```python
from build123d import *

# Parameters (mm, degrees)
BOSS_EXTRUDE2_START = 5
SKETCH6_R           = 3
BOSS_EXTRUDE2_DEPTH = 5


with BuildPart() as part:
    # Sketch2 → Revolve1 (revolve)
    with BuildSketch(Plane.XY, mode=Mode.PRIVATE) as revolve1_sk:
        Polygon((-42.375, 0), (42.375, 0), (42.375, 3), (36.175, 3), (36.175, 3.5), (30.375, 3.5), (30.375, 5), (28.375, 5), (28.375, 6), (-17.625, 6), (-17.625, 5), (-32.375, 5), (-32.375, 3), (-42.375, 3), align=None)
    revolve(revolve1_sk.sketch.rotate(Axis((-42.375, 0, 0), (1, 0, 0)), 90), axis=Axis((-42.375, 0, 0), (1, 0, 0)))

    # Sketch6 → Boss-Extrude2 (add)
    with BuildSketch(Plane.ZY.offset(42.375).offset(BOSS_EXTRUDE2_START)):
        Circle(SKETCH6_R)
    extrude(amount=-BOSS_EXTRUDE2_DEPTH)


solid = part.part
```
CAD build for the part. Positions are in the model's coordinates, mm. A direction names the side the tool comes from. Round coordinates to 2 decimals unless told otherwise and drop trailing zeros. Write each loop counter-clockwise with the first axis right and the second up, starting at its lowest first coordinate (ties: lowest second). Pieces come first, ordered by that corner, then holes. Notation, with made-up numbers: (37.25, 58) -> (89.25, 58) arc R31 ccw to (89.25, 85) -> close; hole circle Ø7 at (20, 80). An arc over 180 degrees is marked (long way). Answer in a Markdown table with one row per item. Add a question column.
Item 1: Saw through at C-C, the plane x = 22.5. Write the cut outline in (y, z).
Item 2: Saw through at A-A, the plane z = 0. Write the cut outline in (x, y) (3 decimals), then the cut area to 3 significant figures.
Item 3: Which spindle directions (+Z, -Z, +X, -X, +Y, -Y) get a long thin tool onto all of the face, cutting with end or side? Do faces 1 (the face through (-32.375, -0.1, 3.3)), 2 (the face through (5.053, -1.802, 5.723)), 3 (the face through (30.375, 3.3, -2.2)). Say none if no direction does.
Item 4: Saw through at D-D, the plane z = 4.25. Write the cut outline in (x, y) (3 decimals), then the cut area to 3 significant figures.
Item 5: Drop flat-ended pins along their axis: pin 1 Ø1 at (x, y) = (0.5, -2) entering from -Z; pin 2 Ø6 at (y, z) = (3, -2.5) entering from -X (3 decimals); pin 3 Ø1.5 at (x, z) = (-24, 1.5) entering from +Y; pin 4 Ø6 at (x, z) = (-28.5, -4) entering from -Y. Give the stop position or say it passes through.
Item 6: Drill centre lines: line 1 (Z direction, x = -19.5, y = 4); line 2 (X direction, y = -4.25, z = -0.5) (3 decimals); line 3 (X direction, y = -5.5, z = 1.25) (3 decimals). Where is each one in solid material? Low to high. Write a range as from..to.
Findings below:
| question | item | result |
|---|---|---|
| 1 | outline | circle Ø12 at (0, 0) |
| 2 | outline | (-47.375, -3) -> (-32.375, -3) -> (-32.375, -5) -> (-17.625, -5) -> (-17.625, -6) -> (28.375, -6) -> (28.375, -5) -> (30.375, -5) -> (30.375, -3.5) -> (36.175, -3.5) -> (36.175, -3) -> (42.375, -3) -> (42.375, 3) -> (36.175, 3) -> (36.175, 3.5) -> (30.375, 3.5) -> (30.375, 5) -> (28.375, 5) -> (28.375, 6) -> (-17.625, 6) -> (-17.625, 5) -> (-32.375, 5) -> (-32.375, 3) -> (-47.375, 3) -> close |
| 2 | area | 887 mm^2 |
| 3 | face 1 | -X |
| 3 | face 2 | +X, -X |
| 3 | face 3 | +X |
| 4 | outline | (-32.375, -2.634) -> (-17.625, -2.634) -> (-17.625, -4.235) -> (28.375, -4.235) -> (28.375, -2.634) -> (30.375, -2.634) -> (30.375, 2.634) -> (28.375, 2.634) -> (28.375, 4.235) -> (-17.625, 4.235) -> (-17.625, 2.634) -> (-32.375, 2.634) -> close |
| 4 | area | 478 mm^2 |
| 5 | pin 1 | stops at z = -5.81 |
| 5 | pin 2 | stops at x = -47.375 |
| 5 | pin 3 | stops at y = 4.94 |
| 5 | pin 4 | stops at y = -4.9 |
| 6 | line 1 | z = -3..3 |
| 6 | line 2 | x = -32.375..30.375 |
| 6 | line 3 | x = -17.625..28.375 |
